The model under review builds one solid part; all positions refer to its coordinate system, in mm. Face numbers are marked on the shaded views. A direction names the side the tool comes from. Coordinates: 2 decimals unless noted, no trailing zeros. Loops run counter-clockwise (first coordinate to the right, second up) from the corner with the lowest first, then second, coordinate; pieces in that order, holes last. Notation, with made-up numbers: (73.25, 76) - (89.25, 76) arc R12 ccw to (89.25, 97) - close; hole circle Ø2 at (39.5, 42). An arc over 180 degrees is marked (long way). Use a Markdown table: item, result. Add a question column.
1) Clearance check with flat-ended pins moving along their axes: pin 1 (2 mm diameter, centred on x = 2.5, z = 2, fed in from +Y); pin 2 (1.5 mm diameter, centred on x = 5, z = 1.5, fed in from -Y); pin 3 (1 mm diameter, centred on x = 4.5, y = -1, fed in from +Z). State where each tip first meets the part, or that it passes through.
2) To check wall thickness, follow L1, parallel to X at y = -0.8, z = 0.6; L2, parallel to Y at x = 0.55, z = -0.95; L3, parallel to Z at x = 4.25, y = 0.2. State the ranges of each line that lie inside material, in increasing order. Write a range as [from, to].
3) The part is to be moulded in two halves that separate along Y. For the marked faces 1, 2 and 3, say which applies: pulls with the +Y half, pulls with the -Y half, needs draft (parallel to the pull), parting line crosses it, or undercut.
4) Add section B-B, the plane z = 0. Give the boundary of the cut face in (x, y).
5) For the marked faces 4, 5 and 6, list the 3-axis set-ups (+Z, -Z, +X, -X, +Y, -Y) from which the entire face can be reached by the end or side of a thin tool; tool diameter is ignored.
6) Add section C-C, the plane x = 3.5. Give the boundary of the cut face in (y, z).
7) Add section A-A, the plane x = 0.55. Give the boundary of the cut face in (y, z).
Autodesk Inventor part; units mm, degrees
ref_plane "YZ Plane" through (0, 0, 0) normal (1, 0, 0) x (0, 1, 0)
ref_plane "XZ Plane" through (0, 0, 0) normal (0, 1, 0) x (-1, 0, 0)
ref_plane "XY Plane" through (0, 0, 0) normal (0, 0, 1) x (1, 0, 0)
sketch "スケッチ1" plane through (0, 0, 0) normal (0, 0, 1) x (1, 0, 0)
  line L0 (0, 0) -> (0, 3)
  line L1 (0, 3) -> (0.2, 3)
  line L2 (0.2, 3) -> (1.7, 1.5)
  line L3 (1.7, 1.5) -> (5.7, 1.5)
  line L4 (5.7, 1.5) -> (5.7, 0)
  line L5 (0, 0) -> (5.7, 0)
  dimension "d0" = 45
  dimension "d1" = 3
  dimension "d2" = 1.7
  dimension "d3" = 1.5
  dimension "d4" = 4
revolve "回転1" add sketch "スケッチ1" angle 360 about axis through (0, 0, 0) along (1, 0, 0)
thread "ねじ1"
sketch "スケッチ2" plane through (0, 0, 0) normal (-1, 0, 0) x (0, 0, 1)
  line L0 (0.5774, 1) -> (1.1547, 0)
  line L1 (1.1547, 0) -> (0.5774, -1)
  line L2 (0.5774, -1) -> (-0.5774, -1)
  line L3 (-0.5774, -1) -> (-1.1547, 0)
  line L4 (-1.1547, 0) -> (-0.5774, 1)
  line L5 (-0.5774, 1) -> (0.5774, 1)
  circle A0 centre (0, 0) radius 1.1547
  point P0 (0, 0)
  point P1 (0, 0)
  dimension "d8" = 2
extrude "押し出し1" cut sketch "スケッチ2" against normal blind 1.2 contours L0 L1 L2 L3 L4 L5
chamfer "面取り1" distance 0.05 angle 45 6 edges at (0, -0.5, -0.866) (0, 0.5, -0.866) (0, 1, 0) (0, 0.5, 0.866) (0, -1, 0) (0, -0.5, 0.866)
chamfer "面取り2" distance 0.15 angle 45 1 edges at (5.7, -1.5, 0)
properties part number "ネジ皿M3L4" material "鋼、高強度、低合金"
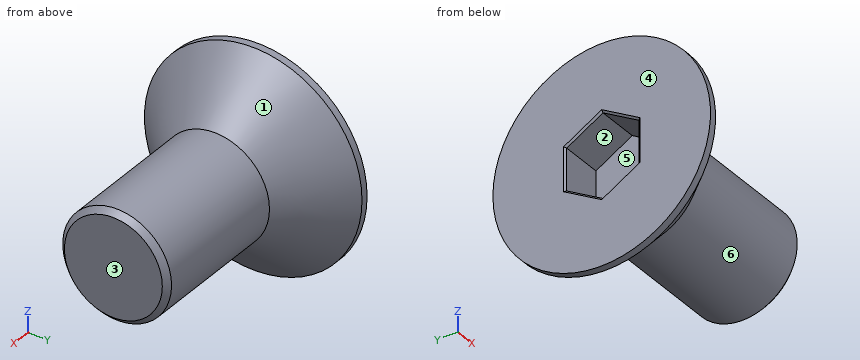
From the geometry:
| question | item | result |
|---|---|---|
| 1 | pin 1 | stops at y = 1.12 |
| 1 | pin 2 | stops at y = -1.3 |
| 1 | pin 3 | stops at z = 1.41 |
| 2 | L1 | x = [1.2, 5.7] |
| 2 | L2 | y = [-2.47, -0.35], [0.35, 2.47] |
| 2 | L3 | z = [-1.49, 1.49] |
| 3 | face 1 | parting line crosses it |
| 3 | face 2 | undercut |
| 3 | face 3 | needs draft |
| 4 | outline | (0, -3) - (0.2, -3) - (1.7, -1.5) - (5.55, -1.5) - (5.7, -1.35) - (5.7, 1.35) - (5.55, 1.5) - (1.7, 1.5) - (0.2, 3) - (0, 3) - (0, 1.05) - (0.05, 1) - (1.2, 1) - (1.2, -1) - (0.05, -1) - (0, -1.05) - close |
| 5 | face 4 | +Z, -Z, -X, +Y, -Y |
| 5 | face 5 | -X |
| 5 | face 6 | +X |
| 6 | outline | circle Ø3 at (0, 0) |
| 7 | outline | circle Ø5.3 at (0, 0); hole (-1, -0.58) - (0, -1.15) - (1, -0.58) - (1, 0.58) - (0, 1.15) - (-1, 0.58) - close |
